```python
from build123d import *

# Parameters (mm, degrees)
BOSS_EXTRUDE1_DEPTH     = 5
BOSS_EXTRUDE2_DEPTH     = 1
SKETCH2_R               = 1.35
CUT_EXTRUDE1_DEPTH      = 39
BOSS_EXTRUDE3_START     = -6
SKETCH3_W               = 3
SKETCH3_H               = 10
BOSS_EXTRUDE3_DEPTH     = 20
BOSS_EXTRU_1_DEPTH      = 4
BOSS_EXTRU_2_DEPTH      = 4
ESQUISSE2_R             = 4.1
ENL_V_MAT_EXTRU_1_DEPTH = 3


with BuildPart() as part:
    # Sketch1 → Boss-Extrude1 (new body)
    with BuildSketch(Plane(origin=(0, 0, 0), x_dir=(1, 0, 0), z_dir=(0, 1, 0))):
        Polygon((2.5, 0), (0, 0), (0, 25), (2.5, 25), (2.5, 31.5), (-2.5, 31.5), (-2.5, -6.5), (2.5, -6.5), align=None)
        Polygon((0, 25), (0, 0), (2.5, 0), (2.5, 4), (2.5, 21), (2.5, 25), align=None)
        Polygon((32.26, 14.5), (2.5, 25), (2.5, 21), (26.591428571, 12.5), align=None)
        Polygon((26.591428571, 12.5), (32.26, 10.5), (37.928571429, 12.5), (32.26, 14.5), align=None)
        Polygon((32.26, 14.5), (37.928571429, 12.5), (62.02, 21), (62.02, 25), align=None)
        Polygon((2.5, 4), (2.5, 0), (32.26, 10.5), (26.591428571, 12.5), align=None)
        Polygon((32.26, 10.5), (62.02, 0), (62.02, 4), (37.928571429, 12.5), align=None)
        Polygon((64.52, 0), (62.02, 0), (62.02, -6.5), (67.02, -6.5), (67.02, 31.5), (62.02, 31.5), (62.02, 25), (64.52, 25), align=None)
        Polygon((62.02, 4), (62.02, 0), (64.52, 0), (64.52, 25), (62.02, 25), (62.02, 21), align=None)
    extrude(amount=BOSS_EXTRUDE1_DEPTH)

    # Sketch1<3> → Boss-Extrude2 (add)
    with BuildSketch(Plane(origin=(0, 0, 0), x_dir=(1, 0, 0), z_dir=(0, 1, 0))):
        Polygon((0, 25), (0, 0), (2.5, 0), (2.5, 4), (2.5, 21), (2.5, 25), align=None)
        Polygon((2.5, 0), (0, 0), (0, 25), (2.5, 25), (2.5, 31.5), (-2.5, 31.5), (-2.5, -6.5), (2.5, -6.5), align=None)
        Polygon((62.02, 4), (62.02, 0), (64.52, 0), (64.52, 25), (62.02, 25), (62.02, 21), align=None)
        Polygon((64.52, 0), (62.02, 0), (62.02, -6.5), (67.02, -6.5), (67.02, 31.5), (62.02, 31.5), (62.02, 25), (64.52, 25), align=None)
    extrude(amount=-BOSS_EXTRUDE2_DEPTH)

    # Sketch2 → Cut-Extrude1 (cut, through all)
    with BuildSketch(Plane(origin=(0, 0, -31.5), x_dir=(-1, 0, 0), z_dir=(0, 0, -1))):
        with Locations((0, 2)):
            Circle(SKETCH2_R)
        with Locations((-64.52, 2)):
            Circle(SKETCH2_R)
    extrude(amount=-CUT_EXTRUDE1_DEPTH, mode=Mode.SUBTRACT)

    # Sketch3 → Boss-Extrude3 (add)
    with BuildSketch(Plane(origin=(0, -1, 0), x_dir=(-1, 0, 0), z_dir=(0, -1, 0)).offset(BOSS_EXTRUDE3_START)):
        with Locations((1, -1.5)):
            Rectangle(SKETCH3_W, SKETCH3_H)
        with Locations((-65.52, -1.5)):
            Rectangle(SKETCH3_W, SKETCH3_H)
    extrude(amount=-BOSS_EXTRUDE3_DEPTH)

    # Sketch4 → Boss.-Extru.1 (add)
    with BuildSketch(Plane(origin=(0, 25, 0), x_dir=(-1, 0, 0), z_dir=(0, -1, 0))):
        Polygon((-0.5, -6.5), (-32.26, -2.5), (-64.02, -6.5), (-67.02, -6.5), (-67.02, 3.5), (-64.02, 3.5), (-32.26, -0.5), (-0.5, 3.5), (2.5, 3.5), (2.5, -6.5), align=None)
        Polygon((-0.5, 1.5), (-24.32, -1.5), (-0.5, -4.5), align=None, mode=Mode.SUBTRACT)
        Polygon((-40.2, -1.5), (-64.02, -4.5), (-64.02, 1.5), align=None, mode=Mode.SUBTRACT)
    extrude(amount=-BOSS_EXTRU_1_DEPTH)

    # Esquisse1 → Boss.-Extru.2 (add)
    with BuildSketch(Plane(origin=(0, 29, 0), x_dir=(1, 0, 0), z_dir=(0, 1, 0))):
        with BuildLine():
            Line((26.092050584, -6.5), (38.427949416, -6.5))
            ThreePointArc((38.427949416, -6.5), (32.26, 6.44), (26.092050584, -6.5))
        make_face()
    extrude(amount=-BOSS_EXTRU_2_DEPTH)

    # Esquisse2 → Enlèv. mat.-Extru.1 (cut)
    with BuildSketch(Plane(origin=(0, 29, 0), x_dir=(1, 0, 0), z_dir=(0, 1, 0))):
        with Locations((32.26, -1.5)):
            Circle(ESQUISSE2_R)
    extrude(amount=-ENL_V_MAT_EXTRU_1_DEPTH, mode=Mode.SUBTRACT)


solid = part.part
```
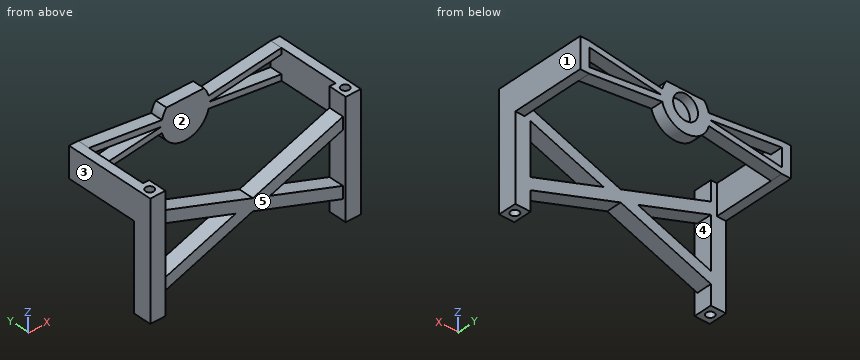
Check sheet for the modelled part. Datum: model origin and axes. Units: mm. Face numbers are marked on the shaded views. A direction names the side the tool comes from. Round coordinates to 2 decimals unless told otherwise and drop trailing zeros. Loops run counter-clockwise (first coordinate to the right, second up) from the corner with the lowest first, then second, coordinate; pieces in that order, holes last. Notation, with made-up numbers: (35.5, 25.25) - (45.5, 25.25) arc R23 ccw to (45.5, 59.25) - close; hole circle Ø2 at (-17.5, 44). An arc over 180 degrees is marked (long way). Answer as a JSON object with one key per item and string values. Group by question number.
Q1. Mould release check, pull along X, two halves, no side actions. Record for the marked faces 1, 2 and 3: released by +X, released by -X, zero draft, split by the parting line, or undercut.
Q2. Sectioned sample at C-C, the plane z = -17. Enter the section's corners in (x, y).
Q3. Scan lines: line 1 along X through (y, z) = (20, -2); line 2 along Y through (x, z) = (64.52, -18.5); line 3 along Y through (x, z) = (0, -1.5). Record each from-to range of solid material in increasing order. Write a range as [from, to].
Q4. Set-up check for the marked faces 4 and 5: record each of +Z, -Z, +X, -X, +Y, -Y from which the full face is reachable in a straight line by a thin tool's end or side.
Q5. Gauge pin test, flat ends, axial feed: P1, Ø4, axis at x = 21.5, z = -14.5, coming from the -Y side; P2, Ø1.5, axis at x = -1.5, y = 22.5, coming from the -Z side; P3, Ø8, axis at y = 12.5, z = -18, coming from the +X side; P4, Ø12, axis at x = 29, y = 4.5, coming from the +Z side. Record the tip position at first contact, or that the pin passes through.
Q6. Sectioned sample at D-D, the plane y = 12. Enter the section's corners in (x, z).
Q7. Sectioned sample at B-B, the plane z = -28. Enter the section's corners in (x, y).
Q8. Sectioned sample at A-A, the plane y = 2. Enter the section's corners in (x, z).
Solution:
{
 "1": {"face 1": "released by +X", "face 2": "undercut", "face 3": "released by -X"},
 "2": {"outline": "(-2.5, -1) - (2.5, -1) - (2.5, 5) - (-2.5, 5) - close; (13.84, 0) - (25.17, 0) - (25.17, 5) - (13.84, 5) - close; (39.35, 0) - (50.68, 0) - (50.68, 5) - (39.35, 5) - close; (62.02, -1) - (67.02, -1) - (67.02, 5) - (62.02, 5) - close; hole circle Ø2.7 at (0, 2); hole circle Ø2.7 at (64.52, 2)"},
 "3": {"line 1": "x = [-2.5, 0.5], [64.02, 67.02]", "line 2": "y = [-1, 0.65], [3.35, 5]", "line 3": "y = [-1, 0.65], [3.35, 29]"},
 "4": {"face 4": "-Y", "face 5": "+Z, -Z, -Y"},
 "5": {"P1": "stops at y = 0", "P2": "stops at z = -3.5", "P3": "passes through", "P4": "stops at z = -7.23"},
 "6": {"outline": "(-2.5, -3.5) - (0.5, -3.5) - (0.5, 6.5) - (-2.5, 6.5) - close; (64.02, -3.5) - (67.02, -3.5) - (67.02, 6.5) - (64.02, 6.5) - close"},
 "7": {"outline": "(-2.5, -1) - (2.5, -1) - (2.5, 5) - (-2.5, 5) - close; (62.02, -1) - (67.02, -1) - (67.02, 5) - (62.02, 5) - close; hole circle Ø2.7 at (0, 2); hole circle Ø2.7 at (64.52, 2)"},
 "8": {"outline": "(-2.5, -31.5) - (-1.35, -31.5) - (-1.35, 6.5) - (-2.5, 6.5) - close; (1.35, -31.5) - (2.5, -31.5) - (2.5, -25) - (32.26, -14.5) - (62.02, -25) - (62.02, -31.5) - (63.17, -31.5) - (63.17, 6.5) - (62.02, 6.5) - (62.02, 0) - (32.26, -10.5) - (2.5, 0) - (2.5, 6.5) - (1.35, 6.5) - close; (65.87, -31.5) - (67.02, -31.5) - (67.02, 6.5) - (65.87, 6.5) - close; hole (2.5, -21) - (26.59, -12.5) - (2.5, -4) - close; hole (37.93, -12.5) - (62.02, -21) - (62.02, -4) - close"}
}
